Part model, mm, in its own coordinate system. Coordinates: 2 decimals unless noted, no trailing zeros. Order: outer loops, then holes, each group sorted by start corner. A loop starts at its lowest first (then second) coordinate and runs counter-clockwise, first axis right, second up.
from build123d import *

# Parameters (mm, degrees)
EXTRUDE018_DEPTH                          = 25.4
EXTRUDE018_ONTO_SKETCH024_PLACEMENT_ANGLE = 8
SKETCH018_AS_DRAWN_R                      = 1.2
EXTRUDE009_DEPTH                          = 7.8
EXTRUDE009_ONTO_SKETCH018_PLACEMENT_ANGLE = 8
EXTRUDE012_DEPTH                          = 6.35
EXTRUDE012_ONTO_SKETCH021_PLACEMENT_ANGLE = 8


with BuildPart() as reset_switch_hole:
    # Sketch024 as drawn → Extrude018 (new, symmetric)
    with BuildSketch(Plane.XY):
        Polygon((-152.83455, 73.27651), (-140.412076, 70.636031), (-143.052554, 58.213557), (-155.475029, 60.854035), align=None)
    extrude(amount=EXTRUDE018_DEPTH, both=True)


with BuildPart() as reset_switch_hole_1:
    # Extrude018 onto Sketch024 placement: moved
    add(reset_switch_hole.part.moved(Location((-7.384231, 0, 52.541536))).rotate(Axis((-7.384231, 0, 52.541536), (0, -1, 0)), EXTRUDE018_ONTO_SKETCH024_PLACEMENT_ANGLE))


with BuildPart() as screw_hole_cuts:
    # Sketch018 as drawn → Extrude009 (new)
    with BuildSketch(Plane.XY):
        with Locations((-31.998318, 84.649891)):
            Circle(SKETCH018_AS_DRAWN_R)
        with Locations((-31.998318, -89.695043)):
            Circle(SKETCH018_AS_DRAWN_R)
        with Locations((156.654735, -49.595599)):
            Circle(SKETCH018_AS_DRAWN_R)
        with Locations((156.654735, 84.649891)):
            Circle(SKETCH018_AS_DRAWN_R)
    extrude(amount=EXTRUDE009_DEPTH)


with BuildPart() as screw_hole_cuts_1:
    # Extrude009 onto Sketch018 placement: moved
    add(screw_hole_cuts.part.moved(Location((39.98734, 0, 30.691416))).rotate(Axis((39.98734, 0, 30.691416), (0, 1, 0)), EXTRUDE009_ONTO_SKETCH018_PLACEMENT_ANGLE))


with BuildPart() as right_top_solid_w_screw_holes:
    # Sketch021 as drawn → Extrude012 (new)
    with BuildSketch(Plane.XY):
        Polygon((-39.826537, 91.531891), (-39.826537, -98.44048), (161.021837, -55.74884), (163.536735, -52.643218), (163.536735, 88.356895), (160.361736, 91.531891), align=None)
    extrude(amount=EXTRUDE012_DEPTH)


with BuildPart() as right_top_solid_w_screw_holes_1:
    # Extrude012 onto Sketch021 placement: moved
    add(right_top_solid_w_screw_holes.part.moved(Location((40.182182, 0, 32.077791))).rotate(Axis((40.182182, 0, 32.077791), (0, 1, 0)), EXTRUDE012_ONTO_SKETCH021_PLACEMENT_ANGLE))

    # Cut004: cut Screw Hole Cuts
    add(screw_hole_cuts_1.part, mode=Mode.SUBTRACT)


with BuildPart() as cut013:
    # Part__Mirroring002: instance of Right Top Solid w/ Screw Holes
    add(right_top_solid_w_screw_holes_1.part.mirror(Plane(origin=(0, 0, 0), x_dir=(0, -1, 0), z_dir=(1, 0, 0))))

    # Cut013: cut Reset Switch Hole
    add(reset_switch_hole_1.part, mode=Mode.SUBTRACT)


solid = cut013.part
Q1. Cut at B-B on y = -28.5. Write the cut outline in (x, z).
Results list:
outline: (-203.01, 15.61) - (-202.13, 9.32) - (-0.74, 37.62) - (-1.63, 43.91) - close
Q2. Pin check, flat tips, straight feed: pin 1 Ø10 at (x, z) = (-156.5, 29) entering from +Y; pin 2 Ø2 at (x, y) = (-177.5, -5) entering from -Z; pin 3 Ø12 at (x, z) = (-83.5, 21.5) entering from -Y. Stop position of each tip, or through.
Results list:
pin 1: passes through
pin 2: stops at z = 12.64
pin 3: stops at y = -81.4
Q3. Cut at C-C on z = 26. Write the cut outline in (x, y).
Results list:
outline: (-129.05, -71.09) - (-83.43, -80.69) - (-83.43, 91.53) - (-129.05, 91.53) - close
Q4. Wall check: line 1 along Z through (x, y) = (-91.5, 63); line 2 along Z through (x, y) = (-127.5, 50.5); line 3 along Y through (x, z) = (-89, 26). Give the ranges that are in metal, low to high.
Results list:
line 1: z = 24.87 to 31.28
line 2: z = 19.81 to 26.22
line 3: y = -79.52 to 91.53
Q5. Cut at A-A on x = -152.5. Write the cut outline in (y, z), and give its area (3 significant figures).
Results list:
outline: (-66.06, 22.7) - (-65.87, 16.29) - (59.42, 16.29) - (59.23, 22.7) - close; (72.22, 22.7) - (72.41, 16.29) - (91.53, 16.29) - (91.53, 22.7) - close
area: 927 mm2
Q6. Mould opens along X. For faces 1 (the face through (-100.909, -2.124, 29.956)), 2 (the face through (-158.32, 66.98, 18.73)), 3 (the face through (-102, 91.532, 27)) say: pulls with the +X half, pulls with the -X half, needs draft (parallel to the pull), parting line crosses it, or undercut.
Results list:
face 1: pulls with the -X half
face 2: undercut
face 3: needs draft
